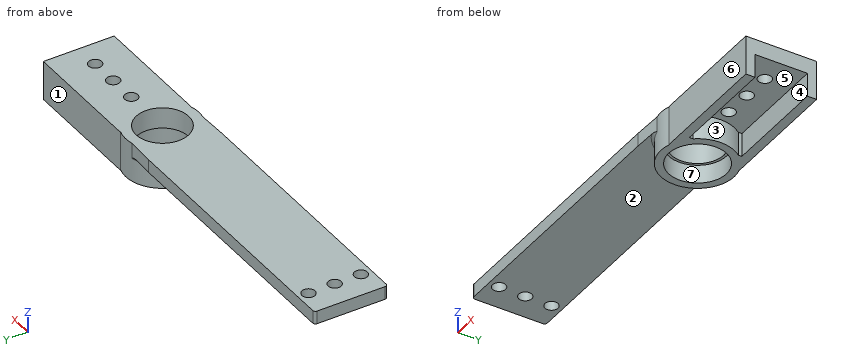
from build123d import *

# Parameters (mm, degrees)
SKETCH_1_W          = 40
SKETCH_1_H          = 20
EXTRUDE_1_DEPTH     = 6
SKETCH_2_R          = 2.5
CUT_EXTRUDE_1_DEPTH = 24.151673806
EXTRUDE_START       = -15
EXTRUDE_2_OUTLINE_R = 11
EXTRUDE_2_DEPTH     = 15
EXTRUDE_START_2     = -8
SKETCH_5_R          = 11
SKETCH_5_R_2        = 10
EXTRUDE_3_DEPTH     = 8
EXTRUDE_START_3     = -5
SKETCH_8_W          = 101
SKETCH_8_H          = 28
EXTRUDE_4_DEPTH     = 5
FILLET_1_R          = 1
FILLET_2_R          = 1
SKETCH_9_R          = 2.5
CUT_EXTRUDE_2_DEPTH = 5


# Read off the part's stored shape, not the designer's step: the extrude step
with BuildPart() as part:
    # Sketch 1 → Extrude 1 (new body)
    with BuildSketch(Plane.XY):
        Rectangle(SKETCH_1_W, SKETCH_1_H)
    extrude(amount=EXTRUDE_1_DEPTH)

    # Sketch 2 → Cut-Extrude 1 (cut, through all)
    with BuildSketch(Plane.XY.offset(6)):
        with Locations((10, 0)):
            Circle(SKETCH_2_R)
        with Locations((-1, 0)):
            Circle(SKETCH_2_R)
        with Locations((-12, 0)):
            Circle(SKETCH_2_R)
    extrude(amount=-CUT_EXTRUDE_1_DEPTH, mode=Mode.SUBTRACT)

    # Extrude 2 outline → Extrude 2 (add)
    with BuildSketch(Plane.XY.offset(6).offset(EXTRUDE_START)):
        with BuildLine():
            Line((20, 10), (20, 13.5))
            Line((20, 13.5), (-26.893967141, 13.5))
            Line((-26.893967141, 13.5), (-26.893967141, 13.384337644))
            ThreePointArc((-26.893967141, 13.384337644), (-45, 0), (-26.893967141, -13.384337644))
            Line((-26.893967141, -13.384337644), (-26.893967141, -13.5))
            Line((-26.893967141, -13.5), (20, -13.5))
            Line((20, -13.5), (20, -10))
            Line((20, -10), (-20, -10))
            Line((-20, -10), (-20, -8.660254038))
            ThreePointArc((-20, -8.660254038), (-17, 0), (-20, 8.660254038))
            Line((-20, 8.660254038), (-20, 10))
            Line((-20, 10), (20, 10))
        make_face()
        with Locations((-31, 0)):
            Circle(EXTRUDE_2_OUTLINE_R, mode=Mode.SUBTRACT)
    extrude(amount=EXTRUDE_2_DEPTH)

    # Sketch 5 → Extrude 3 (add)
    with BuildSketch(Plane.XY.offset(6).offset(EXTRUDE_START_2)):
        with Locations((-31, 0)):
            Circle(SKETCH_5_R)
        with Locations((-31, 0)):
            Circle(SKETCH_5_R_2, mode=Mode.SUBTRACT)
    extrude(amount=EXTRUDE_3_DEPTH)

    # Sketch 8 → Extrude 4 (add)
    with BuildSketch(Plane.XY.offset(6).offset(EXTRUDE_START_3)):
        with Locations((-95.5, 0)):
            Rectangle(SKETCH_8_W, SKETCH_8_H)
        with BuildLine():
            Line((-45, 5.1e-08), (-45, -14))
            Line((-45, -14), (-33.911999365, -13.693803697))
            ThreePointArc((-33.911999365, -13.693803697), (-41.880440979, -8.809994557), (-45, 5.1e-08))
        make_face()
        with BuildLine():
            Line((-45, 14), (-45, 5.1e-08))
            ThreePointArc((-45, 5.1e-08), (-41.968667344, 8.699904408), (-34.187380521, 13.632336755))
            Line((-34.187380521, 13.632336755), (-45, 14))
        make_face()
    extrude(amount=EXTRUDE_4_DEPTH)

    # Fillet 1
    fillet_1_edges = [part.edges().sort_by_distance(p)[0] for p in [
        (-44.999289152, -0.141078849, 1),
    ]]
    fillet(fillet_1_edges, radius=FILLET_1_R)

    # Fillet 2
    fillet_2_edges = [part.edges().sort_by_distance(p)[0] for p in [
        (-146, -14, 3.5),
        (-146, 14, 3.5),
    ]]
    fillet(fillet_2_edges, radius=FILLET_2_R)

    # Sketch 9 → Cut-Extrude 2 (cut)
    with BuildSketch(Plane.XY.offset(6)):
        with Locations((-136, 0)):
            Circle(SKETCH_9_R)
        with Locations((-136, 10)):
            Circle(SKETCH_9_R)
        with Locations((-136, -10)):
            Circle(SKETCH_9_R)
    extrude(amount=-CUT_EXTRUDE_2_DEPTH, mode=Mode.SUBTRACT)


solid = part.part
Check sheet for the modelled part. Datum: model origin and axes. Units: mm. Face numbers are marked on the shaded views. A direction names the side the tool comes from. Round coordinates to 2 decimals unless told otherwise and drop trailing zeros. Order: outer loops, then holes, each group sorted by start corner. A loop starts at its lowest first (then second) coordinate and runs counter-clockwise, first axis right, second up. Notation, with made-up numbers: M 60.25,68 L 105.25,68 A25 ccw 105.25,90 Z; hole C 28.5,30.25 d10. An arc over 180 degrees is marked long. One line per item, written item: value. Start each with the question number.
1. Section check B-B on z = -6.75. Enter the section's corners in (x, y), and give its area (3 significant figures).
2. Section check A-A on x = -31. Enter the section's corners in (y, z).
3. Section check D-D on x = 6. Enter the section's corners in (y, z), and give its area (3 significant figures).
4. Access from +Z, -Z, +X, -X, +Y, -Y to the whole of each face (thin tool, end or side, straight path). Record for the marked faces 5, 6 and 7.
5. Release check for a two-part mould opening along Y. For the marked faces 1, 2, 3 and 4 record: released by +Y, released by -Y, zero draft, split by the parting line, or undercut.
6. Section check C-C on x = -136. Enter the section's corners in (y, z).
7. Scan lines: line 1 along Y through (x, z) = (-136, 3.45); line 2 along Y through (x, z) = (10, 3.5); line 3 along X through (y, z) = (-2.25, 2). Record each from-to range of solid material in increasing order.
8. Gauge pin test, flat ends, axial feed: P1, Ø3, axis at x = -32, z = 0.5, coming from the -Y side; P2, Ø10, axis at x = 7.5, y = -3.5, coming from the -Z side; P3, Ø6.5, axis at x = -136, y = 10, coming from the -Z side; P4, Ø7, axis at x = 2, z = -2.5, coming from the -Y side. Record the tip position at first contact, or that the pin passes through.
Results found:
1. outline: M -26.89,-13.5 L 20,-13.5 L 20,-10 L -20,-10 L -20,-8.66 A14 ccw -20,8.66 L -20,10 L 20,10 L 20,13.5 L -26.89,13.5 L -26.89,13.38 A14 ccw long -26.89,-13.38 Z; hole C -31,0 d22
1. area: 543 mm^2
2. outline: M -14,-9 L -11,-9 L -11,-2 L -10,-2 L -10,6 L -14,6 Z; M 10,-2 L 11,-2 L 11,-9 L 14,-9 L 14,6 L 10,6 Z
3. outline: M -13.5,-9 L -10,-9 L -10,0 L 10,0 L 10,-9 L 13.5,-9 L 13.5,6 L -13.5,6 Z
3. area: 225 mm^2
4. face 5: -Z, +X
4. face 6: +Z, -Z, +X, -Y
4. face 7: -Z
5. face 1: released by +Y
5. face 2: zero draft
5. face 3: undercut
5. face 4: undercut
6. outline: M -14,1 L -12.5,1 L -12.5,6 L -14,6 Z; M -7.5,1 L -2.5,1 L -2.5,6 L -7.5,6 Z; M 2.5,1 L 7.5,1 L 7.5,6 L 2.5,6 Z; M 12.5,1 L 14,1 L 14,6 L 12.5,6 Z
7. line 1: -14 to -12.5, -7.5 to -2.5, 2.5 to 7.5, 12.5 to 14
7. line 2: -13.5 to -2.5, 2.5 to 13.5
7. line 3: -146 to -137.09, -134.91 to -40.74, -21.26 to -13.09, -10.91 to -2.09, 0.09 to 8.91, 11.09 to 20
8. P1: y = -14
8. P2: z = 0
8. P3: z = 1
8. P4: y = -13.5
